The listing builds one solid part. Answer for the finished solid, in the listing's coordinates (mm). A direction names the side the tool comes from. Give positions to 0.01 mm unless a question says otherwise; leave off trailing zeros. Write each loop counter-clockwise with the first axis right and the second up, starting at its lowest first coordinate (ties: lowest second). Pieces come first, ordered by that corner, then holes. Notation, with made-up numbers: (23.25, -30) - (51.25, -30) arc R20 cw to (51.25, 2) - close; hole circle Ø6 at (50, 85). An arc over 180 degrees is marked (long way). Return JSON: item names as keys, results as strings.
from build123d import *

# Parameters (mm, degrees)
F0_W     = 26
F0_H     = 35.5
F1_DEPTH = 7
F4_D     = 4
F5_DEPTH = 10
F7_D     = 4


with BuildPart() as f1:
    # F0 (on Top) → F1 (new body)
    with BuildSketch(Plane.XY):
        Polygon((-46.6139434278, 112), (-61.6139434278, 112), (-61.6139434278, -6.3780904748), (78.3860565722, -6.3780904748), (78.3860565722, 112), (-1.6139434278, 112), (-1.6139434278, 102), (2.3860565722, 102), (2.3860565722, 0), (-51.6139434278, 0), (-51.6139434278, 102), (-46.6139434278, 102), align=None)
        Polygon((13.2124200463, 4.5), (13.2124200463, 36.5), (19.2124200463, 36.5), (19.2124200463, 46.5), (34.2124200463, 46.5), (34.2124200463, 36.5), (39.2124200463, 36.5), (39.2124200463, 4.5), align=None, mode=Mode.SUBTRACT)
        with Locations((50.3860565722, 74.25)):
            Rectangle(F0_W, F0_H, mode=Mode.SUBTRACT)
    extrude(amount=F1_DEPTH)

    # F4 (through all)
    with Locations(Plane.XY.offset(7)):
        with Locations((74.3860565722, 108), (-57.6139434278, 108), (-57.6139434278, 116), (74.3860565722, 116)):
            Hole(F4_D / 2)

    # F5 (add): a face of the model
    f5_faces = [f1.faces().sort_by_distance(p)[0] for p in [
        (-61.6139434278, 52.8109547626, 3.5),
    ]]
    extrude(f5_faces, amount=F5_DEPTH)

    # F7 (through all)
    with Locations(Plane.XY.offset(7)):
        with Locations((-67.6139434278, 109.0609547626), (-67.6139434278, 52.8109547626), (-67.6139434278, -3.4390452374)):
            Hole(F7_D / 2)


solid = f1.part
Item 1: Consider L1, parallel to X at y = 76, z = 2.5; L2, parallel to X at y = 23.5, z = 6; L3, parallel to Y at x = -51, z = 6.5. Determine where each line is inside the solid, lowest interval first.
Answer below:
{"L1": "x = -71.61 to -51.61, 2.39 to 37.39, 63.39 to 78.39", "L2": "x = -71.61 to -51.61, 2.39 to 13.21, 39.21 to 78.39", "L3": "y = -6.38 to 0, 102 to 112"}
Item 2: A cutting plane is placed at B-B on y = 59. Determine the outline of the cut face in (x, z), then the cut area to 3 significant figures.
Answer below:
{"outline": "(-71.61, 0) - (-51.61, 0) - (-51.61, 7) - (-71.61, 7) - close; (2.39, 0) - (37.39, 0) - (37.39, 7) - (2.39, 7) - close; (63.39, 0) - (78.39, 0) - (78.39, 7) - (63.39, 7) - close", "area": "490 mm²"}
Item 3: A cutting plane is placed at A-A on x = 31. Determine the outline of the cut face in (y, z).
Answer below:
{"outline": "(-6.38, 0) - (4.5, 0) - (4.5, 7) - (-6.38, 7) - close; (46.5, 0) - (112, 0) - (112, 7) - (46.5, 7) - close"}
Item 4: For faces 1 (the face through (19.212, 41, 3)), 2 (the face through (-1.614, 107, 3)), 3 (the face through (21, 54, 7)), determine the directions among +Z, -Z, +X, -X, +Y, -Y from which every point of the face is accessible in a straight line to the end or side of a thin tool.
Answer below:
{"face 1": "+Z, -Z", "face 2": "+Z, -Z, +Y", "face 3": "+Z, +X, -X, +Y, -Y"}
Item 5: A cutting plane is placed at D-D on x = -24. Determine the outline of the cut face in (y, z), then the cut area to 3 significant figures.
Answer below:
{"outline": "(-6.38, 0) - (0, 0) - (0, 7) - (-6.38, 7) - close", "area": "44.6 mm²"}
Item 6: The mould has two halves that part along X. Classify faces 4 (the face through (4, -6.378, 3)), 5 (the face through (78.386, 52, 3)), 6 (the face through (16, 36.5, 3)): +X half, -X half, draft (parallel to the pull), parting line (faces both ways), or undercut.
Answer below:
{"face 4": "draft", "face 5": "+X half", "face 6": "undercut"}
Item 7: A cutting plane is placed at C-C on z = 2. Give the number of separate pieces and of enclosed holes in the cut face, then the cut area to 3 significant figures.
Answer below:
{"separate pieces": "1", "enclosed holes": "7", "area": "9,830 mm²"}
